Source: CAD feature listing. Evaluate the final solid. Frame: model axes, mm. Face numbers are marked on the shaded views. Round coordinates to 2 decimals unless told otherwise and drop trailing zeros. Loops run counter-clockwise (first coordinate to the right, second up) from the corner with the lowest first, then second, coordinate; pieces in that order, holes last. Notation, with made-up numbers: M -0.75,-37.75 L 41.25,-37.75 A28 cw 41.25,-4.75 Z; hole C 66,73 d3. An arc over 180 degrees is marked long. Answer as a JSON object with one key per item and string values.
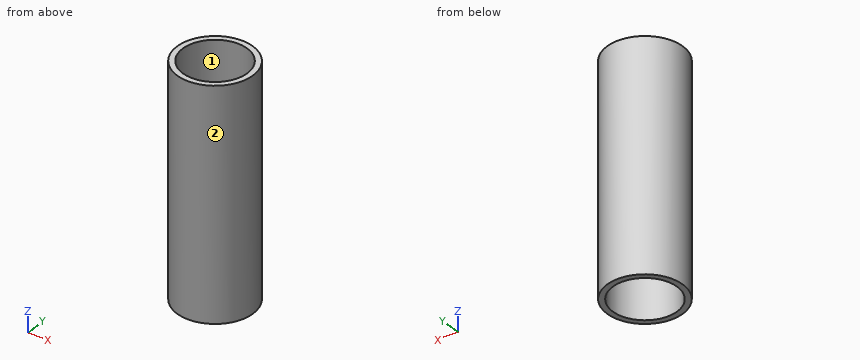
from build123d import *

# Parameters (mm, degrees)
F0_R      = 12.7
F1_DEPTH  = 50.8
F1_FACE_R = 12.7
F2_DEPTH  = 25.4
F4_D      = 21.59


with BuildPart() as f1:
    # F0 (on Top) → F1 (new body)
    with BuildSketch(Plane.XY):
        Circle(F0_R)
    extrude(amount=F1_DEPTH)

    # F1_face (on face) → F2 (join)
    with BuildSketch(Plane.XY.offset(50.8)):
        Circle(F1_FACE_R)
    extrude(amount=F2_DEPTH)

    # F4 (through all)
    with Locations(Plane.XY.offset(76.2)):
        with Locations((0, 0)):
            Hole(F4_D / 2)


solid = f1.part
Item 1: Line query: probe 1 along Y at (x, z) = (0, 59.5) (3 decimals); probe 2 along Y at (x, z) = (4.5, 71); probe 3 along X at (y, z) = (-5.25, 16.5). Output: solid intervals per line, ascending. Write a range as from..to.
Answer sheet:
{"probe 1": "y = -12.7..-10.795, 10.795..12.7", "probe 2": "y = -11.88..-9.81, 9.81..11.88", "probe 3": "x = -11.56..-9.43, 9.43..11.56"}
Item 2: Section C-C on z = 43.5. Return the cut outline in (x, y) (3 decimals), then the cut area to 3 significant figures.
Answer sheet:
{"outline": "C 0,0 d25.4; hole C 0,0 d21.59", "area": "141 mm²"}
Item 3: Section A-A on y = 0. Return the cut outline in (x, z) (3 decimals).
Answer sheet:
{"outline": "M -12.7,0 L -10.795,0 L -10.795,76.2 L -12.7,76.2 Z; M 10.795,0 L 12.7,0 L 12.7,76.2 L 10.795,76.2 Z"}
Item 4: Pull-direction query (Y, two-part tool) for the marked faces 1 and 2; classes: pulls with the +Y half, pulls with the -Y half, needs draft (parallel to the pull), parting line crosses it, or undercut.
Answer sheet:
{"face 1": "undercut", "face 2": "parting line crosses it"}
Item 5: Contact query for flat-ended pins moving along their axis: pin 1 Ø5 at (x, y) = (2.5, 8) entering from +Z; pin 2 Ø8 at (x, z) = (8, 48.5) entering from -Y; pin 3 Ø3 at (y, z) = (-2.5, 16) entering from +X; pin 4 Ø12 at (y, z) = (-8, 50.5) entering from -X. Output: stop coordinate, or through.
Answer sheet:
{"pin 1": "stops at z = 76.2", "pin 2": "stops at y = -12.05", "pin 3": "stops at x = 12.66", "pin 4": "stops at x = -12.54"}
